from build123d import *

# Parameters (mm, degrees)
SKETCH1_W            = 16.31
SKETCH1_H            = 16.31
SKETCH1_R            = 4.5
BOSS_EXTRUDE1_DEPTH  = 4
SKETCH3_R            = 1.5
CUT_EXTRUDE1_DEPTH   = 4
BOSS_EXTRUDE2_DEPTH  = 4
BOSS_EXTRUDE6_DEPTH  = 4
CUT_EXTRUDE3_DEPTH   = 4
BOSS_EXTRUDE7_DEPTH  = 4
BOSS_EXTRUDE9_DEPTH  = 4
SKETCH17_OUTSIDE_W   = 136.165
SKETCH17_OUTSIDE_H   = 117.232
CUT_EXTRUDE4_DEPTH   = 4
SKETCH18_R           = 1.5
BOSS_EXTRUDE10_DEPTH = 4
CUT_EXTRUDE5_DEPTH   = 4
SKETCH20_R           = 2
CUT_EXTRUDE6_DEPTH   = 10
SKETCH22_R           = 1.75
CUT_EXTRUDE8_DEPTH   = 124.744497459


with BuildPart() as part:
    # Sketch1 → Boss-Extrude1 (new body)
    with BuildSketch(Plane(origin=(0, 0, 0), x_dir=(1, 0, 0), z_dir=(0, 1, 0))):
        Rectangle(SKETCH1_W, SKETCH1_H)
        with Locations(Location((0, 0, 0), (0, 0, 270))):
            Circle(SKETCH1_R, mode=Mode.SUBTRACT)
    extrude(amount=BOSS_EXTRUDE1_DEPTH)

    # Sketch3 → Cut-Extrude1 (cut)
    with BuildSketch(Plane(origin=(0, 4, 0), x_dir=(1, 0, 0), z_dir=(0, 1, 0))):
        with Locations(Location((5.656854249, 5.656854249, 0), (0, 0, 270))):
            Circle(SKETCH3_R)
        with Locations(Location((5.656854249, -5.656854249, 0), (0, 0, 270))):
            Circle(SKETCH3_R)
        with Locations(Location((-5.656854249, -5.656854249, 0), (0, 0, 270))):
            Circle(SKETCH3_R)
        with Locations(Location((-5.656854249, 5.656854249, 0), (0, 0, 270))):
            Circle(SKETCH3_R)
    extrude(amount=-CUT_EXTRUDE1_DEPTH, mode=Mode.SUBTRACT)

    # Sketch4 → Boss-Extrude2 (add)
    with BuildSketch(Plane(origin=(0, 4, 0), x_dir=(1, 0, 0), z_dir=(0, 1, 0))):
        Polygon((8.155, -8.155), (0, -8.155), (0, -10.655), (10.655, -10.655), (10.655, 0), (8.155, 0), align=None)
    extrude(amount=-BOSS_EXTRUDE2_DEPTH)

    # Sketch9 → Boss-Extrude6 (add)
    with BuildSketch(Plane(origin=(0, 4, 0), x_dir=(1, 0, 0), z_dir=(0, 1, 0))):
        Polygon((71.061407011, -58.982568069), (7.593139788, -10.281653748), (10.613791504, -4.032054751), (84.193483815, -43.982568069), (90.501950314, -50.291034568), (96.061407011, -50.291034568), (96.061407011, -73.982568069), (81.061407011, -73.982568069), (81.061407011, -68.982568069), align=None)
    extrude(amount=-BOSS_EXTRUDE6_DEPTH)

    # Sketch12 → Cut-Extrude3 (cut)
    with BuildSketch(Plane(origin=(0, 4, 0), x_dir=(1, 0, 0), z_dir=(0, 1, 0))):
        Polygon((87.278639473, -47.258318902), (85.780514725, -48.583317861), (89.960889469, -52.761034568), (90.501950314, -52.761034568), (96.061407011, -52.761034568), (96.061407011, -50.291034568), (90.501950314, -50.291034568), (87.347717064, -47.136801318), align=None)
    extrude(amount=-CUT_EXTRUDE3_DEPTH, mode=Mode.SUBTRACT)

    # Sketch13 → Boss-Extrude7 (add)
    with BuildSketch(Plane(origin=(0, 4, 0), x_dir=(1, 0, 0), z_dir=(0, 1, 0))):
        Polygon((81.061407011, -73.982568069), (81.061407011, -77.282568069), (96.561407011, -77.282568069), (96.561407011, -52.761034568), (96.061407011, -52.761034568), (96.061407011, -73.982568069), align=None)
    extrude(amount=-BOSS_EXTRUDE7_DEPTH)

    # Sketch16 → Boss-Extrude9 (add)
    with BuildSketch(Plane(origin=(0, 4, 0), x_dir=(1, 0, 0), z_dir=(0, 1, 0))):
        Polygon((0, -10.655), (-10, -10.655), (-10, 10.345), (10.655, 10.345), (10.655, 0), (8.155, 0), (8.155, 8.155), (-8.155, 8.155), (-8.155, -8.155), (0, -8.155), align=None)
    extrude(amount=-BOSS_EXTRUDE9_DEPTH)

    # Sketch17 outside → Cut-Extrude4 (cut)
    with BuildSketch(Plane(origin=(0, 4, 0), x_dir=(1, 0, 0), z_dir=(0, 1, 0))):
        with Locations((43.2805, -33.469)):
            Rectangle(SKETCH17_OUTSIDE_W, SKETCH17_OUTSIDE_H)
        with BuildLine():
            Line((5.656854249, -8.656854249), (5.656854249, -10.655))
            Line((5.656854249, -10.655), (8.079694096, -10.655))
            Line((8.079694096, -10.655), (71.061407011, -58.982568069))
            Line((71.061407011, -58.982568069), (81.061407011, -68.982568069))
            Line((81.061407011, -68.982568069), (81.061407011, -77.282568069))
            Line((81.061407011, -77.282568069), (96.561407011, -77.282568069))
            Line((96.561407011, -77.282568069), (96.561407011, -52.761034568))
            Line((96.561407011, -52.761034568), (89.960889469, -52.761034568))
            Line((89.960889469, -52.761034568), (85.780514725, -48.583317861))
            Line((85.780514725, -48.583317861), (87.278639473, -47.258318902))
            Line((87.278639473, -47.258318902), (84.193483815, -43.982568069))
            Line((84.193483815, -43.982568069), (10.655, -4.054429139))
            Line((10.655, -4.054429139), (8.656854249, -5.656854249))
            ThreePointArc((8.656854249, -5.656854249), (6.313708499, 0), (8.656854249, 5.656854249))
            ThreePointArc((8.656854249, 5.656854249), (8.656854249, 8.656854249), (5.656854249, 8.656854249))
            ThreePointArc((5.656854249, 8.656854249), (0, 6.313708499), (-5.656854249, 8.656854249))
            ThreePointArc((-5.656854249, 8.656854249), (-8.656854249, 8.656854249), (-8.656854249, 5.656854249))
            ThreePointArc((-8.656854249, 5.656854249), (-6.313708499, 0), (-8.656854249, -5.656854249))
            ThreePointArc((-8.656854249, -5.656854249), (-8.656854249, -8.656854249), (-5.656854249, -8.656854249))
            ThreePointArc((-5.656854249, -8.656854249), (0, -6.313708499), (5.656854249, -8.656854249))
        make_face(mode=Mode.SUBTRACT)
    extrude(amount=-CUT_EXTRUDE4_DEPTH, mode=Mode.SUBTRACT)

    # Sketch18 → Boss-Extrude10 (add)
    with BuildSketch(Plane(origin=(0, 4, 0), x_dir=(1, 0, 0), z_dir=(0, 1, 0))):
        Polygon((5.656854249, -10.655), (0, -6.313708499), (6.372805828, -0.97060021), (10.655, -4.054429139), (8.656854249, -5.656854249), align=None)
        with Locations(Location((5.656854249, -5.656854249, 0), (0, 0, 270))):
            Circle(SKETCH18_R, mode=Mode.SUBTRACT)
    extrude(amount=-BOSS_EXTRUDE10_DEPTH)

    # Sketch19 → Cut-Extrude5 (cut)
    with BuildSketch(Plane(origin=(0, 4, 0), x_dir=(1, 0, 0), z_dir=(0, 1, 0))):
        with BuildLine():
            Line((97.061407011, -77.355955856), (97.061407011, -59.355955856))
            ThreePointArc((97.061407011, -59.355955856), (93.061407011, -61.012810105), (89.061407011, -59.355955856))
            ThreePointArc((89.061407011, -59.355955856), (92.789329073, -68.355955856), (89.061407011, -77.355955856))
            Line((89.061407011, -77.355955856), (97.061407011, -77.355955856))
        make_face()
    extrude(amount=-CUT_EXTRUDE5_DEPTH, mode=Mode.SUBTRACT)

    # Sketch20 → Cut-Extrude6 (cut)
    with BuildSketch(Plane.XZ):
        with Locations(Location((81.807805677, 62.103797793, 0), (0, 0, 270))):
            Circle(SKETCH20_R)
    extrude(amount=-CUT_EXTRUDE6_DEPTH, mode=Mode.SUBTRACT)

    # Sketch22 → Cut-Extrude8 (cut, through all)
    with BuildSketch(Plane.XZ):
        with Locations(Location((85.097804106, 72.282568069, 0), (0, 0, 270))):
            Circle(SKETCH22_R)
    extrude(amount=-CUT_EXTRUDE8_DEPTH, mode=Mode.SUBTRACT)


solid = part.part
Design review of the part built by this model. Coordinates are the model's own, in mm. A direction names the side the tool comes from. Give positions to 0.01 mm unless a question says otherwise; leave off trailing zeros. Loops run counter-clockwise (first coordinate to the right, second up) from the corner with the lowest first, then second, coordinate; pieces in that order, holes last. Notation, with made-up numbers: M 61.5,-6 L 100.5,-6 A14 cw 100.5,9 Z; hole C 89,59 d11. An arc over 180 degrees is marked long. Write item = value, one per line.
Q1. For faces 1 (the cylindrical face through (-6.314, 2.028, -0.088)), 2 (the flat face through (87.8, 2, 50.6)), 3 (the cylindrical face through (-8.624, 2.028, -8.689)), 4 (the flat face through (2.868, 2.028, 8.515)), 5 (the flat face through (7, 2, 10.655)), list the 3-axis set-ups (+Z, -Z, +X, -X, +Y, -Y) from which the entire face can be reached by the end or side of a thin tool; tool diameter is ignored.
Output values:
face_1 = -X, +Y, -Y
face_2 = +X, +Y, -Y
face_3 = +Y, -Y
face_4 = +Z, +Y, -Y
face_5 = +Z, -X, +Y, -Y
Q2. Draft analysis for pull direction Z (two halves, no side actions). For faces 6 (the flat face through (93, 2, 52.761)), 7 (the cylindrical face through (1.352, 1.972, 4.292)), 8 (the flat face through (76.13, 2.03, 64.05)), state which applies: +Z half, -Z half, draft (parallel to the pull), parting line (faces both ways), or undercut.
Output values:
face_6 = -Z half
face_7 = undercut
face_8 = +Z half
Q3. Insertion check: pin 1 (2 mm diameter, centred on x = 75.5, y = 2.5, fed in from +Z); pin 2 (3 mm diameter, centred on x = 81.81, z = 62.1, fed in from -Y); pin 3 (1.5 mm diameter, centred on y = 0.5, z = 41.5, fed in from +X); pin 4 (1.9 mm diameter, centred on x = 6.5, y = 1.5, fed in from +Z) (3 decimals). Each pin has a flat end and moves straight along its axis. Give the tip position at first contact, or say it passes through.
Output values:
pin_1 = 64.42
pin_2 = through
pin_3 = 81
pin_4 = 10.655
Q4. We need section C-C (z = 22.5). Give the boundary of the cut face in (x, y), plus the area to 3 significant figures.
Output values:
outline = M 23.52,0 L 44.63,0 L 44.63,4 L 23.52,4 Z
area = 84.4 mm^2
Q5. We need section A-A (y = 3.15). Count the separate pieces of the cut face and the enclosed holes in it, plus the area to 3 significant figures.
Output values:
separate_pieces = 1
enclosed_holes = 7
area = 1,680 mm^2
Q6. We need section B-B (x = 46). Give the boundary of the cut face in (y, z).
Output values:
outline = M 0,23.25 L 4,23.25 L 4,39.75 L 0,39.75 Z
Q7. To check wall thickness, follow line 1 (X direction, y = 3.5, z = 72.5); line 2 (Z direction, x = 38, y = 3.85); line 3 (Z direction, x = 10, y = 3.45). State the ranges of each line that lie inside material, in increasing order. Write a range as [from, to].
Output values:
line_1 = [81.06, 83.36], [86.83, 92.1]
line_2 = [18.9, 33.61]
line_3 = [3.58, 12.13]
